Answer from the drawing. Dimensions are ordinates in mm from the lowest x, y and z of the part. A direction names the side the tool comes from. Give positions to 0.01 mm unless a question says otherwise; leave off trailing zeros. Loops run counter-clockwise (first coordinate to the right, second up) from the corner with the lowest first, then second, coordinate; pieces in that order, holes last.
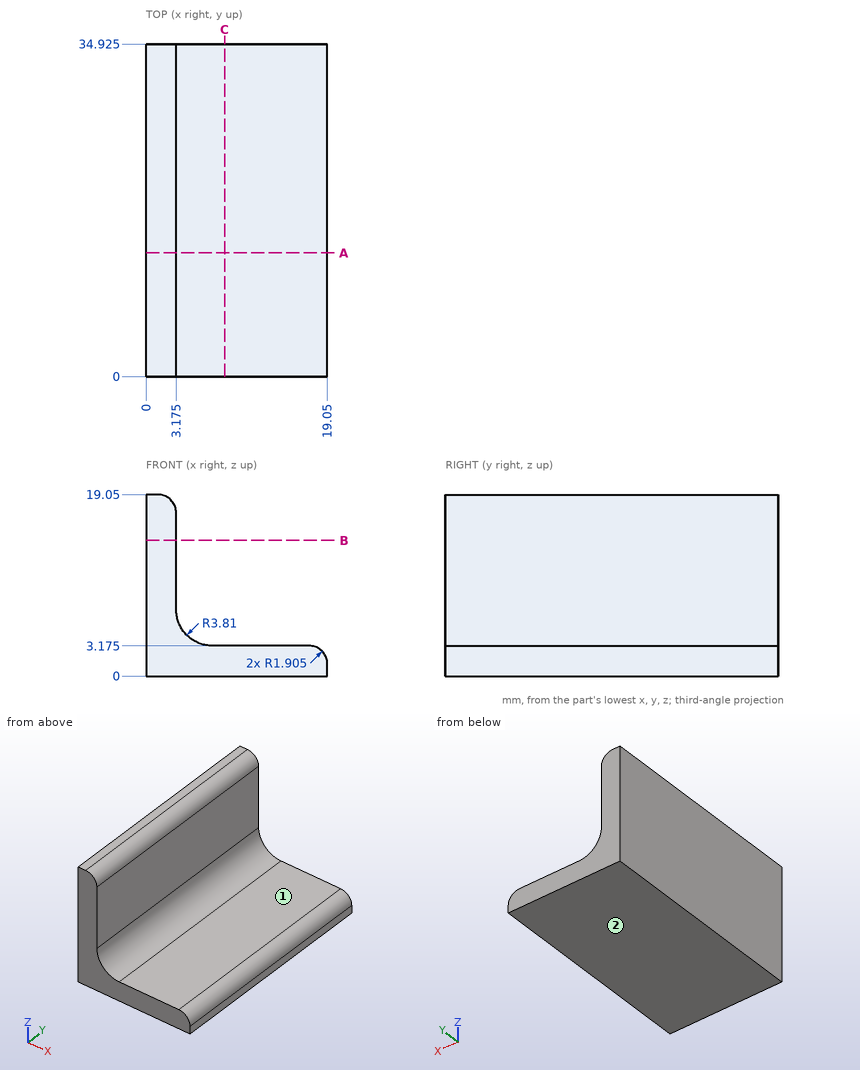
Item 1: Find section C-C, the plane x = 8.25. Write down the section's boundary in (y, z) (3 decimals).
Item 2: Flat-ended cylindrical pins translate along their axes: pin 1 Ø1 at (y, z) = (30, 4) entering from -X; pin 2 Ø1.5 at (x, y) = (11.5, 16.5) entering from +Z (3 decimals); pin 3 Ø8 at (y, z) = (17, 10.5) entering from +X; pin 4 Ø1.5 at (y, z) = (18.5, 3.5) entering from +X. Find the tip coordinate at first contact, or state that the pin passes through.
Item 3: Find section A-A, the plane y = 13. Write down the section's boundary in (x, z) (3 decimals).
Item 4: Consider line 1 (X direction, y = 2, z = 15.25) (3 decimals); line 2 (Z direction, x = 3.75, y = 19.5). Determine where each line is inside the solid, lowest interval first.
Item 5: Find section B-B, the plane z = 14.25. Write down the section's boundary in (x, y) (3 decimals), plus the area to 3 significant figures.
Item 6: For the marked faces 1 and 2, determine the directions among +Z, -Z, +X, -X, +Y, -Y from which every point of the face is accessible in a straight line to the end or side of a thin tool.
Ans:
1. outline: (0, 0) - (34.925, 0) - (34.925, 3.175) - (0, 3.175) - close
2. pin 1: stops at x = 0
2. pin 2: stops at z = 3.175
2. pin 3: stops at x = 3.21
2. pin 4: stops at x = 18.34
3. outline: (0, 0) - (19.05, 0) - (19.05, 1.27) arc R1.905 ccw to (17.145, 3.175) - (6.985, 3.175) arc R3.81 cw to (3.175, 6.985) - (3.175, 17.145) arc R1.905 ccw to (1.27, 19.05) - (0, 19.05) - close
4. line 1: x = 0 to 3.175
4. line 2: z = 0 to 4.97
5. outline: (0, 0) - (3.175, 0) - (3.175, 34.925) - (0, 34.925) - close
5. area: 111 mm2
6. face 1: +Z, +X, +Y, -Y
6. face 2: -Z, +X, -X, +Y, -Y
